from build123d import *

# Parameters (mm, degrees)
SKETCH1_R           = 3
SKETCH1_R_2         = 1.5
BOSS_EXTRUDE1_DEPTH = 6


with BuildPart() as part:
    # Sketch1 → Boss-Extrude1 (new body)
    with BuildSketch(Plane.XY):
        with BuildLine():
            Line((0, 35), (168.284271247, 35))
            ThreePointArc((168.284271247, 35), (172.111105571, 34.238795325), (175.355339059, 32.071067812))
            Line((175.355339059, 32.071067812), (191.213203436, 16.213203436))
            ThreePointArc((191.213203436, 16.213203436), (186.901061777, -29.786167732), (142.50454583, -17))
            ThreePointArc((142.50454583, -17), (135.128694201, -8.266799469), (124.17424305, -5))
            Line((124.17424305, -5), (48.989794856, -5))
            ThreePointArc((48.989794856, -5), (38.545135498, -7.943942692), (31.175323999, -15.909090909))
            ThreePointArc((31.175323999, -15.909090909), (-29.84810029, -18.278153875), (0, 35))
        make_face()
        Circle(SKETCH1_R, mode=Mode.SUBTRACT)
        with Locations((50, 15)):
            Circle(SKETCH1_R, mode=Mode.SUBTRACT)
        with Locations((100, 15)):
            Circle(SKETCH1_R, mode=Mode.SUBTRACT)
        with Locations((183.241017493, -11.134594342)):
            Circle(SKETCH1_R_2, mode=Mode.SUBTRACT)
        with Locations((176.134594342, -18.241017493)):
            Circle(SKETCH1_R_2, mode=Mode.SUBTRACT)
        with Locations((141.769204776, 16.124372073)):
            Circle(SKETCH1_R_2, mode=Mode.SUBTRACT)
        with Locations((148.875627927, 23.230795224)):
            Circle(SKETCH1_R_2, mode=Mode.SUBTRACT)
        Polygon((155.434043323, 24.768752473), (184.778974742, -4.576178946), (169.576178946, -19.778974742), (140.231247527, 9.565956677), align=None, mode=Mode.SUBTRACT)
    extrude(amount=BOSS_EXTRUDE1_DEPTH)


solid = part.part
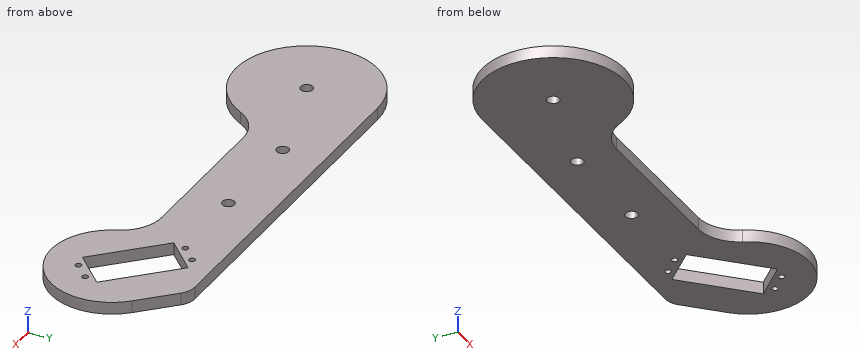
Could you check a few things on this model? Use its own coordinates, in mm. Coordinates: 2 decimals unless noted, no trailing zeros. Loops run counter-clockwise (first coordinate to the right, second up) from the corner with the lowest first, then second, coordinate; pieces in that order, holes last. Notation, with made-up numbers: (-28.75, 38) -> (0.25, 38) arc R17 ccw to (0.25, 43) -> close; hole circle Ø1 at (51, 44.25). An arc over 180 degrees is marked (long way). Answer in a Markdown table with one row per item.
(1) If I drill on probe 1 along Y at (x, z) = (0, 3.6); probe 2 along X at (y, z) = (-0.5, 3); probe 3 along X at (y, z) = (17, 4), over which ranges is the centre line in solid material (lowest first)?
Results found:
| item | result |
|---|---|
| probe 1 | y = -35 to -3, 3 to 35 |
| probe 2 | x = -35 to -2.96, 2.96 to 150.3, 180.7 to 199.66 |
| probe 3 | x = -30.59 to 47.76, 52.24 to 97.76, 102.24 to 140.55, 142.99 to 147.67, 163.2 to 190.43 |
(2) Imagine slicing it at C-C (y = 0). List the corners of the cut face in (x, z) for me, plus the area to 3 significant figures.
Results found:
| item | result |
|---|---|
| outline | (-35, 0) -> (-3, 0) -> (-3, 6) -> (-35, 6) -> close; (3, 0) -> (149.8, 0) -> (149.8, 6) -> (3, 6) -> close; (180.2, 0) -> (199.58, 0) -> (199.58, 6) -> (180.2, 6) -> close |
| area | 1,190 mm^2 |
(3) Imagine slicing it at D-D (z = 4.2). Give the number of separate pieces and of enclosed holes in the cut face, plus the area to 3 significant figures.
Results found:
| item | result |
|---|---|
| separate pieces | 1 |
| enclosed holes | 8 |
| area | 10,800 mm^2 |
(4) Imagine slicing it at B-B (y = -27). List the corners of the cut face in (x, z) for me, plus the area to 3 significant figures.
Results found:
| item | result |
|---|---|
| outline | (-22.27, 0) -> (22.27, 0) -> (22.27, 6) -> (-22.27, 6) -> close; (149.6, 0) -> (190.4, 0) -> (190.4, 6) -> (149.6, 6) -> close |
| area | 512 mm^2 |
(5) Imagine slicing it at A-A (x = 100). List the corners of the cut face in (y, z) for me.
Results found:
| item | result |
|---|---|
| outline | (-5, 0) -> (12, 0) -> (12, 6) -> (-5, 6) -> close; (18, 0) -> (35, 0) -> (35, 6) -> (18, 6) -> close |
(6) Will these pins go through, and if not, where does the flat tip stop? pin 1 Ø8 at (x, y) = (171.5, -12.5) entering from -Z; pin 2 Ø5.5 at (x, y) = (0, 0) entering from +Z.
Results found:
| item | result |
|---|---|
| pin 1 | stops at z = 0 |
| pin 2 | passes through |
